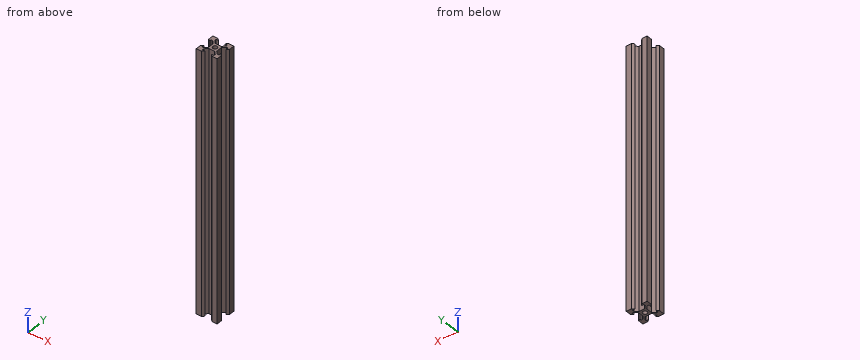
```python
from build123d import *

# Parameters (mm, degrees)
SKETCH1_R           = 2.1
BOSS_EXTRUDE1_DEPTH = 125


with BuildPart() as part:
    # Sketch1 → Boss-Extrude1 (new, symmetric)
    with BuildSketch(Plane.XY):
        Polygon((-10, 10), (-5, 10), (-3.2, 8.2), (-5.499339828, 8.2), (-5.499339828, 6.56), (-2.84, 3.900660172), (2.84, 3.900660172), (5.499339828, 6.56), (5.499339828, 8.2), (3.2, 8.2), (5, 10), (10, 10), (10, 5), (8.2, 3.2), (8.2, 5.499339828), (6.56, 5.499339828), (3.900660172, 2.84), (3.900660172, -2.84), (6.56, -5.499339828), (8.2, -5.499339828), (8.2, -3.2), (10, -5), (10, -10), (5, -10), (3.2, -8.2), (5.499339828, -8.2), (5.499339828, -6.56), (2.84, -3.900660172), (-2.84, -3.900660172), (-5.499339828, -6.56), (-5.499339828, -8.2), (-3.2, -8.2), (-5, -10), (-10, -10), (-10, -5), (-8.2, -3.2), (-8.2, -5.499339828), (-6.56, -5.499339828), (-3.900660172, -2.84), (-3.900660172, 2.84), (-6.56, 5.499339828), (-8.2, 5.499339828), (-8.2, 3.2), (-10, 5), align=None)
        with Locations(Location((0, 0, 0), (0, 0, 180))):
            Circle(SKETCH1_R, mode=Mode.SUBTRACT)
    extrude(amount=BOSS_EXTRUDE1_DEPTH, both=True)


solid = part.part
```
Geometry check sheet. Reference: the model listing, model coordinates, mm. Round coordinates to 2 decimals unless told otherwise and drop trailing zeros. Loops run counter-clockwise (first coordinate to the right, second up) from the corner with the lowest first, then second, coordinate; pieces in that order, holes last. Notation, with made-up numbers: (-15.75, 57.5) - (41.25, 57.5) arc R13 cw to (41.25, 72.5) - close; hole circle Ø5 at (-28, 84.25). An arc over 180 degrees is marked (long way). Write each question's results on one line, items separated by ' | '. Start each with the question number.
Q1. Cross-section at A-A on y = 0. Enter the section's corners in (x, z), and give its area (3 significant figures).
Q2. Thickness scan on line 1 (Y direction, x = 0, z = -14); line 2 (X direction, y = 4.5, z = 102.5); line 3 (X direction, y = 4.25, z = -66). Record the ranges inside material, lowest first. Write a range as [from, to].
Q3. Gauge pin test, flat ends, axial feed: P1, Ø6, axis at y = 1, z = 16.5, coming from the -X side; P2, Ø3, axis at y = 1, z = -78, coming from the +X side; P3, Ø4.5, axis at y = 1, z = 36, coming from the +X side; P4, Ø3, axis at x = 1, y = -6.5, coming from the +Z side. Record the tip position at first contact, or that the pin passes through.
Answers below:
1) outline: (-3.9, -125) - (-2.1, -125) - (-2.1, 125) - (-3.9, 125) - close; (2.1, -125) - (3.9, -125) - (3.9, 125) - (2.1, 125) - close | area: 900 mm²
2) line 1: y = [-3.9, -2.1], [2.1, 3.9] | line 2: x = [-9.5, -8.2], [-5.56, -3.44], [3.44, 5.56], [8.2, 9.5] | line 3: x = [-9.25, -8.2], [-5.31, -3.19], [3.19, 5.31], [8.2, 9.25]
3) P1: stops at x = -9 | P2: stops at x = 3.9 | P3: stops at x = 8.25 | P4: passes through
